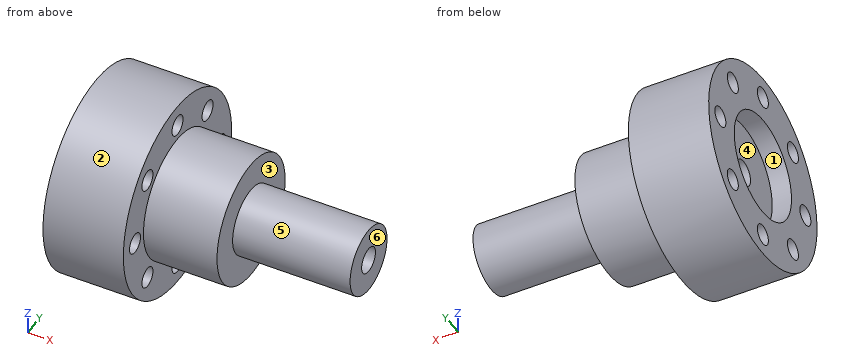
```python
from build123d import *

# Parameters (mm, degrees)
F2_R     = 20.746813
F3_DEPTH = 7.62
F4_R     = 5.02647
F5_DEPTH = 107.404763
F6_R     = 3.988802
F7_DEPTH = 107.404763


with BuildPart() as f1:
    # F0 (on Front) → F1 (revolve)
    with BuildSketch(Plane.XZ):
        Polygon((0, 39.248202), (0, 0), (107.403763, 0), (107.403763, 13.375257), (60.913306, 13.375257), (60.913306, 24.69467), (31.806249, 24.69467), (31.806249, 39.248202), align=None)
    revolve(axis=Axis((53.701881, 0, 0), (-1, 0, 0)))

    # F2 (on face) → F3 (cut)
    with BuildSketch(Plane(origin=(0, 0, 0), x_dir=(0, -1, 0), z_dir=(-1, 0, 0))):
        Circle(F2_R)
    extrude(amount=-F3_DEPTH, mode=Mode.SUBTRACT)

    # F4 (on face) → F5 (cut, through all)
    with BuildSketch(Plane.YZ.offset(107.403763)):
        Circle(F4_R)
    extrude(amount=-F5_DEPTH, mode=Mode.SUBTRACT)

    # F6 (on face) → F7 (cut, through all)
    with BuildSketch(Plane(origin=(0, 0, 0), x_dir=(0, -1, 0), z_dir=(-1, 0, 0))):
        with Locations((0, 30.801583)):
            Circle(F6_R)
        with Locations((-21.780009, 21.780009)):
            Circle(F6_R)
        with Locations((-30.801583, 0)):
            Circle(F6_R)
        with Locations((-21.780009, -21.780009)):
            Circle(F6_R)
        with Locations((0, -30.801583)):
            Circle(F6_R)
        with Locations((21.780009, -21.780009)):
            Circle(F6_R)
        with Locations((30.801583, 0)):
            Circle(F6_R)
        with Locations((21.780009, 21.780009)):
            Circle(F6_R)
    extrude(amount=-F7_DEPTH, mode=Mode.SUBTRACT)


solid = f1.part
```
Input: part model. Units: mm. Frame: model coordinates. Face numbers are marked on the shaded views. A direction names the side the tool comes from. Give positions to 0.01 mm unless a question says otherwise; leave off trailing zeros. Order: outer loops, then holes, each group sorted by start corner. A loop starts at its lowest first (then second) coordinate and runs counter-clockwise, first axis right, second up. Notation, with made-up numbers: (37.5, -22.75) - (46.5, -22.75) arc R25 cw to (46.5, 16.25) - close; hole circle Ø4 at (38.5, 65.25). An arc over 180 degrees is marked (long way). Use a Markdown table: item, result.
(1) Section query C-C (y = -33.5). Output: boundary loops of the cut face in (x, z), then the cut area to 3 significant figures.
Computed values:
| item | result |
|---|---|
| outline | (0, -20.45) - (31.81, -20.45) - (31.81, -2.94) - (0, -2.94) - close; (0, 2.94) - (31.81, 2.94) - (31.81, 20.45) - (0, 20.45) - close |
| area | 1,110 mm2 |
(2) Pin query (flat end, axial travel): pin 1 (12 mm diameter, centred on x = 69, z = -28, fed in from -Y); pin 2 (3 mm diameter, centred on y = 18.5, z = -2, fed in from -X); pin 3 (5 mm diameter, centred on x = 40, y = -5.5, fed in from +Z); pin 4 (10.5 mm diameter, centred on y = -30.8, z = 0, fed in from +X). Return the tip coordinate at first contact, or that it passes through.
Computed values:
| item | result |
|---|---|
| pin 1 | passes through |
| pin 2 | stops at x = 7.62 |
| pin 3 | stops at z = 24.51 |
| pin 4 | stops at x = 31.81 |
(3) Section query D-D (x = 94). Output: boundary loops of the cut face in (y, z), then the cut area to 3 significant figures.
Computed values:
| item | result |
|---|---|
| outline | circle Ø26.75 at (0, 0); hole circle Ø10.05 at (0, 0) |
| area | 483 mm2 |
(4) Access query for the marked faces 1, 2 and 3. Directions: +Z, -Z, +X, -X, +Y, -Y. A direction counts if a zero-diameter tool reaches every point of the face in a straight line with its end or side. Return the directions, or none.
Computed values:
| item | result |
|---|---|
| face 1 | -X |
| face 2 | +X, -X |
| face 3 | +X |
(5) Section query A-A (y = 0). Output: boundary loops of the cut face in (x, z).
Computed values:
| item | result |
|---|---|
| outline | (0, -39.25) - (31.81, -39.25) - (31.81, -34.79) - (0, -34.79) - close; (0, -26.81) - (31.81, -26.81) - (31.81, -24.69) - (60.91, -24.69) - (60.91, -13.38) - (107.4, -13.38) - (107.4, -5.03) - (7.62, -5.03) - (7.62, -20.75) - (0, -20.75) - close; (0, 20.75) - (7.62, 20.75) - (7.62, 5.03) - (107.4, 5.03) - (107.4, 13.38) - (60.91, 13.38) - (60.91, 24.69) - (31.81, 24.69) - (31.81, 26.81) - (0, 26.81) - close; (0, 34.79) - (31.81, 34.79) - (31.81, 39.25) - (0, 39.25) - close |
(6) Line query: line 1 (X direction, y = 25, z = 18); line 2 (Y direction, x = 80, z = 3); line 3 (X direction, y = -11, z = -13). Output: solid intervals per line, ascending. Write a range as from..to.
Computed values:
| item | result |
|---|---|
| line 1 | x = 0..31.81 |
| line 2 | y = -13.03..-4.03, 4.03..13.03 |
| line 3 | x = 7.62..60.91 |
(7) Draft query along Z for the marked faces 4, 5 and 6. Return one class per face: released by +Z, released by -Z, zero draft, split by the parting line, or undercut.
Computed values:
| item | result |
|---|---|
| face 4 | undercut |
| face 5 | split by the parting line |
| face 6 | zero draft |
